```python
from build123d import *

# Parameters (mm, degrees)
SKETCH072_W          = 62
SKETCH072_H          = 62
PAD012_DEPTH         = 18
SKETCH073_R          = 3.05
POCKET058_DEPTH      = 18.001
POCKET059_DEPTH      = 59
POCKET060_DEPTH      = 7
SKETCH077_R          = 1.5
POCKET062_DEPTH      = 22
SKETCH078_R          = 5.5
POCKET063_DEPTH      = 15
SKETCH076_W          = 31
SKETCH076_H          = 7
SKETCH076_W_2        = 1
SKETCH076_H_2        = 8
POCKET065_DEPTH      = 11
POCKET_DEPTH         = 7
POCKET068_DEPTH      = 31.001
POCKET068_DEPTH_BACK = -31.001
POCKET069_DEPTH      = 16
SKETCH_W             = 6
SKETCH_H             = 2
POCKET070_DEPTH      = 0.2


with BuildPart() as part:
    # Sketch072 → Pad012 (new body)
    with BuildSketch(Plane.XY):
        Rectangle(SKETCH072_W, SKETCH072_H)
    extrude(amount=PAD012_DEPTH)

    # Sketch073 (on Face5 of Pad012) → Pocket058 (cut, through all)
    with BuildSketch(Plane(origin=(0, 0, 0), x_dir=(1, 0, 0), z_dir=(0, 0, -1))):
        with Locations((-25, 25)):
            Circle(SKETCH073_R)
        with Locations((25, 25)):
            Circle(SKETCH073_R)
        with Locations((-25, -25)):
            Circle(SKETCH073_R)
        with Locations((25, -25)):
            Circle(SKETCH073_R)
        Circle(SKETCH073_R)
        with Locations((0, -25)):
            Circle(SKETCH073_R)
    extrude(amount=-POCKET058_DEPTH, mode=Mode.SUBTRACT)

    # Sketch074 (on Face2 of Pocket058) → Pocket059 (cut)
    with BuildSketch(Plane.XZ.offset(31)):
        Polygon((-21.25, 20), (-21.25, 15), (-24.25, 15), (-24.25, 11), (-17.75, 11), (-17.75, 18), (17.75, 18), (17.75, 11), (24.25, 11), (24.25, 15), (21.25, 15), (21.25, 20), align=None)
    extrude(amount=-POCKET059_DEPTH, mode=Mode.SUBTRACT)

    # Sketch075 (on Face5 of Pocket059) → Pocket060 (cut)
    with BuildSketch(Plane.XY.offset(18)):
        Polygon((-19, -11), (-19, 9), (19, 9), (19, -11), (23, -20), (31, -20), (31, -31), (-31, -31), (-31, -20), (-23, -20), align=None)
    extrude(amount=-POCKET060_DEPTH, mode=Mode.SUBTRACT)

    # Sketch077 → Pocket062 (cut)
    with BuildSketch(Plane(origin=(0, 31, 0), x_dir=(-1, 0, 0), z_dir=(0, 1, 0))):
        with Locations((-11, 13.5)):
            Circle(SKETCH077_R)
        with Locations((11, 13.5)):
            Circle(SKETCH077_R)
    extrude(amount=-POCKET062_DEPTH, mode=Mode.SUBTRACT)

    # Sketch078 (on Face4 of Pocket062) → Pocket063 (cut)
    with BuildSketch(Plane.XY.offset(18)):
        with Locations((-25, 25)):
            Circle(SKETCH078_R)
        with Locations((-25, -25)):
            Circle(SKETCH078_R)
        with Locations((25, 25)):
            Circle(SKETCH078_R)
        with Locations((25, -25)):
            Circle(SKETCH078_R)
        Circle(SKETCH078_R)
        with Locations((0, 25)):
            Circle(SKETCH078_R)
    extrude(amount=-POCKET063_DEPTH, mode=Mode.SUBTRACT)

    # Sketch076 (on Face4 of Pocket060) → Pocket065 (cut)
    with BuildSketch(Plane.XY.offset(18)):
        with Locations((0, -23)):
            Rectangle(SKETCH076_W, SKETCH076_H)
        with Locations((-12, 5)):
            Rectangle(SKETCH076_W_2, SKETCH076_H_2)
        with Locations((12, 5)):
            Rectangle(SKETCH076_W_2, SKETCH076_H_2)
    extrude(amount=-POCKET065_DEPTH, mode=Mode.SUBTRACT)

    # Sketch079 → Pocket (cut)
    with BuildSketch(Plane.XY.offset(18)):
        Polygon((-25, 20), (-20, 15), (-20, 25), align=None)
        Polygon((20, 25), (20, 15), (25, 20), align=None)
    extrude(amount=-POCKET_DEPTH, mode=Mode.SUBTRACT)

    # Sketch080 → Pocket068 (cut, two sides)
    with BuildSketch(Plane.YZ) as pocket068_sk:
        Polygon((-31, 11), (-31, 9), (-29, 11), align=None)
    extrude(amount=-POCKET068_DEPTH, mode=Mode.SUBTRACT)
    extrude(pocket068_sk.sketch, amount=-POCKET068_DEPTH_BACK, mode=Mode.SUBTRACT)

    # Sketch081 (on Face44 of Pocket068) → Pocket069 (cut)
    with BuildSketch(Plane.XZ.offset(-9)):
        with BuildLine():
            ThreePointArc((-9, 15), (-11, 17), (-13, 15))
            Line((-13, 15), (-13, 12))
            ThreePointArc((-13, 12), (-11, 10), (-9, 12))
            Line((-9, 15), (-9, 12))
        make_face()
        with BuildLine():
            ThreePointArc((13, 15), (11, 17), (9, 15))
            Line((9, 15), (9, 12))
            ThreePointArc((9, 12), (11, 10), (13, 12))
            Line((13, 15), (13, 12))
        make_face()
    extrude(amount=-POCKET069_DEPTH, mode=Mode.SUBTRACT)

    # Sketch (on Face22 of Pocket069) → Pocket070 (cut)
    with BuildSketch(Plane.XY.offset(18)):
        Polygon((-11, 16), (-13, 16), (-13, 14), (-15, 14), (-15, 12), (-13, 12), (-13, 10), (-11, 10), (-11, 12), (-9, 12), (-9, 14), (-11, 14), align=None)
        with Locations((12, 13)):
            Rectangle(SKETCH_W, SKETCH_H)
    extrude(amount=-POCKET070_DEPTH, mode=Mode.SUBTRACT)


solid = part.part
```
The listing builds one solid part. Answer for the finished solid, in the listing's coordinates (mm). A direction names the side the tool comes from. Give positions to 0.01 mm unless a question says otherwise; leave off trailing zeros. Order: outer loops, then holes, each group sorted by start corner. A loop starts at its lowest first (then second) coordinate and runs counter-clockwise, first axis right, second up. Notation, with made-up numbers: (60.25, -3.75) - (86.25, -3.75) arc R18 cw to (86.25, 6.25) - close; hole circle Ø9 at (22, 0.5). An arc over 180 degrees is marked (long way). Answer in a Markdown table with one row per item. Add a question column.
Q1. The part is cut by section C-C (y = -6.5). Determine the outline of the cut face in (x, z), then the cut area to 4 significant figures.
Q2. Which of the six approach directions +Z, -Z, +X, -X, +Y, -Y give full straight-line access (tool end or side, diameter ignored) to faces 1 (the flat face through (12, 13, 17.8)), 2 (the flat face through (-9, 17, 14)), 3 (the cylindrical face through (11, 17, 10))?
Q3. The part is cut by section A-A (y = -25). Determine the outline of the cut face in (x, z).
Q4. Find the intervals of material crossed by line 1 along X through (y, z) = (25, 1.95); line 2 along X through (y, z) = (7.5, 7.5); line 3 along Y through (x, z) = (2.5, 5.75), in increasing order. Write a range as [from, to].
Q5. Given P1, Ø3, axis at x = -5.5, z = 15.5, coming from the -Y side; P2, Ø1.9, axis at x = 28.5, z = 15, coming from the -Y side; P3, Ø2, axis at x = -3.5, y = -22.5, coming from the +Z side; P4, Ø5, axis at x = 2.5, y = -10.5, coming from the -Z side, each flat-ended and moving along its own axis, determine where each tip first touches the part or whether it passes through.
Q6. The part is cut by section B-B (z = 1.5). Determine the outline of the cut face in (x, y).
Q7. For a pull along X with two mould halves and no side action, classify faces 4 (the flat face through (0, 9, 15)), 5 (the flat face through (0, 31, 9)), 6 (the flat face through (-31, 0, 9)) as released by +X, released by -X, zero draft, split by the parting line, or undercut.
Determined:
| question | item | result |
|---|---|---|
| 1 | outline | (-31, 0) - (31, 0) - (31, 18) - (21.25, 18) - (21.25, 15) - (24.25, 15) - (24.25, 11) - (-24.25, 11) - (-24.25, 15) - (-21.25, 15) - (-21.25, 18) - (-31, 18) - close |
| 1 | area | 794.5 mm² |
| 2 | face 1 | +Z |
| 2 | face 2 | -Y |
| 2 | face 3 | none |
| 3 | outline | (-31, 0) - (-28.05, 0) - (-28.05, 3) - (-30.5, 3) - (-30.5, 11) - (-31, 11) - close; (-21.95, 0) - (21.95, 0) - (21.95, 3) - (19.5, 3) - (19.5, 11) - (15.5, 11) - (15.5, 7) - (-15.5, 7) - (-15.5, 11) - (-19.5, 11) - (-19.5, 3) - (-21.95, 3) - close; (28.05, 0) - (31, 0) - (31, 11) - (30.5, 11) - (30.5, 3) - (28.05, 3) - close |
| 4 | line 1 | x = [-31, -28.05], [-21.95, -3.05], [3.05, 21.95], [28.05, 31] |
| 4 | line 2 | x = [-31, -12.5], [-11.5, 11.5], [12.5, 31] |
| 4 | line 3 | y = [-31, -4.9], [4.9, 20.1], [29.9, 31] |
| 5 | P1 | stops at y = 9 |
| 5 | P2 | stops at y = -20 |
| 5 | P3 | stops at z = 7 |
| 5 | P4 | stops at z = 0 |
| 6 | outline | (-31, -31) - (31, -31) - (31, 31) - (-31, 31) - close; hole circle Ø6.1 at (-25, -25); hole circle Ø6.1 at (-25, 25); hole circle Ø6.1 at (0, 0); hole circle Ø6.1 at (0, 25); hole circle Ø6.1 at (25, -25); hole circle Ø6.1 at (25, 25) |
| 7 | face 4 | undercut |
| 7 | face 5 | zero draft |
| 7 | face 6 | released by -X |
